Verification items for the finished model (mm, model axes). A direction names the side the tool comes from. Round coordinates to 2 decimals unless told otherwise and drop trailing zeros. Loops run counter-clockwise (first coordinate to the right, second up) from the corner with the lowest first, then second, coordinate; pieces in that order, holes last. Notation, with made-up numbers: (32, -0.5) - (90, -0.5) arc R28 cw to (90, 23.5) - close; hole circle Ø6 at (66.5, -31). An arc over 180 degrees is marked (long way). Use CSV: the item, a comma, the result in double quotes.
```python
from build123d import *

# Parameters (mm, degrees)
SKETCH1_W           = 42.42562
SKETCH1_H           = 1
BOSS_EXTRUDE1_DEPTH = 19.99996
FILLET1_R           = 1
SKETCH2_W           = 34.8742
SKETCH2_H           = 17.79996
SKETCH2_W_2         = 32.8742
SKETCH2_H_2         = 15.79996
BOSS_EXTRUDE2_DEPTH = 1.5


with BuildPart() as part:
    # Sketch1 → Boss-Extrude1 (new body)
    with BuildSketch(Plane.XY):
        with Locations((21.21281, 0.5)):
            Rectangle(SKETCH1_W, SKETCH1_H)
    extrude(amount=BOSS_EXTRUDE1_DEPTH)

    # Fillet1
    # the kernel refuses this fillet: 1 mm, written as the material it takes off along each edge
    with BuildSketch(Plane(origin=(41.42562, 1, 18.99996), x_dir=(1, 0, 0), z_dir=(0, -1, 0))) as fillet1_piece_1_section:
        Polygon((0, 0), (FILLET1_R * 1.02, 0), (FILLET1_R * 1.02, FILLET1_R * 1.02), (0, FILLET1_R * 1.02), align=None)
    fillet1_piece_1 = extrude(amount=FILLET1_R * 1.02, mode=Mode.PRIVATE)
    fillet1_piece_1 = fillet1_piece_1 - Plane(origin=(41.42562, 1, 18.99996), x_dir=(-0.7071067811865475, 0, -0.7071067811865475), z_dir=(0, -1, 0)) * Sphere(FILLET1_R, mode=Mode.PRIVATE)
    add(fillet1_piece_1, mode=Mode.SUBTRACT)
    with BuildSketch(Plane(origin=(41.42562, 1, 1), x_dir=(1, 0, 0), z_dir=(0, -1, 0))) as fillet1_piece_2_section:
        Polygon((0, 0), (FILLET1_R * 1.02, 0), (FILLET1_R * 1.02, -FILLET1_R * 1.02), (0, -FILLET1_R * 1.02), align=None)
    fillet1_piece_2 = extrude(amount=FILLET1_R * 1.02, mode=Mode.PRIVATE)
    fillet1_piece_2 = fillet1_piece_2 - Plane(origin=(41.42562, 1, 1), x_dir=(-0.7071067811865475, 0, 0.7071067811865475), z_dir=(0, -1, 0)) * Sphere(FILLET1_R, mode=Mode.PRIVATE)
    add(fillet1_piece_2, mode=Mode.SUBTRACT)
    with BuildSketch(Plane(origin=(-2.5, 0, 0), x_dir=(0, 0, 1), z_dir=(1, 0, 0))) as fillet1_piece_3:
        with BuildLine():
            CenterArc((FILLET1_R, -FILLET1_R), FILLET1_R, 90, 90)
            Line((0, -FILLET1_R), (0, 0))
            Line((0, 0), (FILLET1_R, 0))
        make_face()
    extrude(amount=43.92562, mode=Mode.SUBTRACT)
    with BuildSketch(Plane(origin=(-2.5, 0, 19.99996), x_dir=(0, 0, -1), z_dir=(1, 0, 0))) as fillet1_piece_4:
        with BuildLine():
            CenterArc((FILLET1_R, FILLET1_R), FILLET1_R, 180, 90)
            Line((0, FILLET1_R), (0, 0))
            Line((0, 0), (FILLET1_R, 0))
        make_face()
    extrude(amount=43.92562, mode=Mode.SUBTRACT)
    with BuildSketch(Plane(origin=(42.42562, 0, 1), x_dir=(-1, 0, 0), z_dir=(0, 0, 1))) as fillet1_piece_5:
        with BuildLine():
            CenterArc((FILLET1_R, -FILLET1_R), FILLET1_R, 90, 90)
            Line((0, -FILLET1_R), (0, 0))
            Line((0, 0), (FILLET1_R, 0))
        make_face()
    extrude(amount=17.99996, mode=Mode.SUBTRACT)

    # Sketch2 → Boss-Extrude2 (add)
    with BuildSketch(Plane(origin=(0, 1, 0), x_dir=(1, 0, 0), z_dir=(0, 1, 0))):
        with Locations((23.88852, -9.99998)):
            Rectangle(SKETCH2_W, SKETCH2_H)
        with Locations((23.88852, -9.99998)):
            Rectangle(SKETCH2_W_2, SKETCH2_H_2, mode=Mode.SUBTRACT)
    extrude(amount=BOSS_EXTRUDE2_DEPTH)


solid = part.part
```
1) Cross-section at C-C, the plane x = 9. Record the cut outline in (y, z), then the cut area to 3 significant figures.
Returned:
outline,"(0, 1) arc R1 ccw to (1, 0) - (1, 1.1) - (2.5, 1.1) - (2.5, 2.1) - (1, 2.1) - (1, 17.9) - (2.5, 17.9) - (2.5, 18.9) - (1, 18.9) - (1, 20) arc R1 ccw to (0, 19) - close"
area,"22.6 mm²"
2) Gauge pin test, flat ends, axial feed: pin 1 Ø0.8 at (y, z) = (2, 14) entering from +X; pin 2 Ø1.2 at (x, y) = (27, 2) entering from +Z; pin 3 Ø0.8 at (y, z) = (2, 6) entering from -X. Record the tip position at first contact, or that the pin passes through.
Returned:
pin 1,"stops at x = 41.33"
pin 2,"stops at z = 18.9"
pin 3,"stops at x = 6.45"
3) Access from +Z, -Z, +X, -X, +Y, -Y to the whole of each face (thin tool, end or side, straight path). Record for faces 4 (the face through (6.451, 2, 10)), 5 (the face through (41.326, 2, 10)), 6 (the face through (24, 2, 1.1)), 7 (the face through (24, 1, 10)).
Returned:
face 4,"+Z, -Z, -X, +Y"
face 5,"+Z, -Z, +X, +Y"
face 6,"-Z, +X, -X, +Y"
face 7,"+Y"
4) Cross-section at A-A, the plane z = 6.5. Record the cut outline in (x, y), then the cut area to 3 significant figures.
Returned:
outline,"(0, 0) - (41.43, 0) arc R1 ccw to (42.43, 1) - (41.33, 1) - (41.33, 2.5) - (40.33, 2.5) - (40.33, 1) - (7.45, 1) - (7.45, 2.5) - (6.45, 2.5) - (6.45, 1) - (0, 1) - close"
area,"45.2 mm²"
5) Mould release check, pull along X, two halves, no side actions. Record for faces 1 (the face through (40.326, 2, 10)), 2 (the face through (14.8, 1, 0.3)), 3 (the face through (42.125, 0.285, 9.874)): +X half, -X half, draft (parallel to the pull), parting line (faces both ways), or undercut.
Returned:
face 1,"undercut"
face 2,"draft"
face 3,"+X half"
6) Cross-section at B-B, the plane y = 1.75. Record the cut outline in (x, z), then the cut area to 3 significant figures.
Returned:
outline,"(6.45, 1.1) - (41.33, 1.1) - (41.33, 18.9) - (6.45, 18.9) - close; hole (7.45, 2.1) - (40.33, 2.1) - (40.33, 17.9) - (7.45, 17.9) - close"
area,"101 mm²"
7) Thickness scan on probe 1 along Z at (x, y) = (16.5, 1.55); probe 2 along X at (y, z) = (1.1, 8.25); probe 3 along Y at (x, z) = (23.5, 10). Record the ranges inside material, lowest first. Write a range as [from, to].
Returned:
probe 1,"z = [1.1, 2.1], [17.9, 18.9]"
probe 2,"x = [6.45, 7.45], [40.33, 41.33]"
probe 3,"y = [0, 1]"
